```python
from build123d import *

# Parameters (mm, degrees)
Y_KSEKLIK_EKSTR_ZYON1_DEPTH = 40
BO_ALTMA1_START             = 2
BO_ALTMA1_DEPTH             = 36
IZIM4_W                     = 38.8
IZIM4_H                     = 1.5
KES_EKSTR_ZYON1_DEPTH       = 10
IZIM5_R                     = 1.45
IZIM5_R_2                   = 19
KES_EKSTR_ZYON2_DEPTH       = 2
IZIM6_W                     = 6.5
IZIM6_H                     = 6.5
IZIM6_R                     = 1.55
Y_KSEKLIK_EKSTR_ZYON2_DEPTH = 3
RADYUS1_R                   = 2
KES_EKSTR_ZYON3_DEPTH       = 10
KES_EKSTR_ZYON3_DEPTH_BACK  = 55


# Read off the part's stored shape, not the designer's step: İç Boşaltma1
with BuildPart() as part:
    # Çizim2 → Yükseklik-Ekstrüzyon1 (new body)
    with BuildSketch(Plane(origin=(0, 0, 0), x_dir=(0, 0, -1), z_dir=(1, 0, 0))):
        with BuildLine():
            Line((-8.520601237, 2.655177464), (-8.520601237, -7.344822536))
            ThreePointArc((-8.520601237, -7.344822536), (-8.2732007, -8.537800405), (-7.571803773, -9.53401603))
            Line((-7.571803773, -9.53401603), (-2.399280893, -14.708783566))
            ThreePointArc((-2.399280893, -14.708783566), (-1.426311448, -15.35897725), (-0.27796055, -15.587463223))
            Line((-0.27796055, -15.587463223), (-1.843021011, -18.19863418))
            add(Edge.make_bspline(
                [(-46.665907249, -13.909076506), (-24.516902354, -18.673937552), (-1.843021011, -18.19863418)],
                knots=[0, 0, 0, 1, 1, 1], degree=2))
            Line((-46.665907249, -13.909076506), (-46.665907249, -11.228578501))
            Line((-46.665907249, -11.228578501), (-8.520601237, 2.655177464))
        make_face()
    extrude(amount=Y_KSEKLIK_EKSTR_ZYON1_DEPTH)

    # İç Boşaltma1 outline → İç Boşaltma1 (cut)
    with BuildSketch(Plane.YZ.offset(BO_ALTMA1_START)):
        with BuildLine():
            Line((-0.201118549, 10.520601237), (-12.409947295, 44.064082645))
            add(Edge.make_bspline(
                [(-12.409947295, 44.064082645), (-12.786167702, 42.211926114), (-13.142061282, 40.357797151), (-13.477631026, 38.501688751), (-13.792879631, 36.643593797), (-14.087809503, 34.783505061), (-14.362422751, 32.921415207), (-14.616721192, 31.057316786), (-14.850706351, 29.19120224), (-15.064379456, 27.323063899), (-15.257741445, 25.452893983), (-15.526587368, 22.544304232), (-15.616158228, 21.507298941), (-15.699505521, 20.469667421), (-15.77662923, 19.431408364), (-15.847529338, 18.39252046), (-15.912205827, 17.353002403), (-15.970658681, 16.312852883), (-16.02288788, 15.272070593), (-16.06889341, 14.230654225), (-16.108675251, 13.18860247), (-16.159012454, 11.624569796), (-16.174235562, 11.103066399), (-16.187902686, 10.581403672), (-16.200013803, 10.059581454), (-16.210568888, 9.537599587), (-16.219567918, 9.01545791), (-16.227010868, 8.493156266), (-16.232897715, 7.970694494), (-16.237228434, 7.448072435), (-16.240003003, 6.92528993), (-16.241792402, 6.157267265), (-16.242021612, 5.912152435), (-16.241909023, 5.667002314), (-16.241454632, 5.421816888), (-16.240658436, 5.176596139), (-16.23952043, 4.931340051), (-16.238040611, 4.68604861), (-16.236218976, 4.440721798), (-16.234055521, 4.1953596), (-16.231550242, 3.949961999), (-16.228703137, 3.704528981)],
                knots=[0.04971795, 0.04971795, 0.04971795, 0.04971795, 0.04971795, 0.04971795, 0.04971795, 0.04971795, 0.04971795, 0.04971795, 0.04971795, 0.04971795, 0.513850496, 0.513850496, 0.513850496, 0.513850496, 0.513850496, 0.513850496, 0.513850496, 0.513850496, 0.513850496, 0.513850496, 0.770775744, 0.770775744, 0.770775744, 0.770775744, 0.770775744, 0.770775744, 0.770775744, 0.770775744, 0.770775744, 0.770775744, 0.899238368, 0.899238368, 0.899238368, 0.899238368, 0.899238368, 0.899238368, 0.899238368, 0.899238368, 0.899238368, 0.899238368, 0.959442934, 0.959442934, 0.959442934, 0.959442934, 0.959442934, 0.959442934, 0.959442934, 0.959442934, 0.959442934, 0.959442934, 0.959442934, 0.959442934], degree=11))
            ThreePointArc((-16.228703137, 3.704528981), (-16.17611264, 3.759568607), (-16.122690278, 3.81380118))
            Line((-16.122690278, 3.81380118), (-10.968143105, 8.966112527))
            ThreePointArc((-10.968143105, 8.966112527), (-9.316172777, 10.115574384), (-7.344822536, 10.520601237))
            Line((-7.344822536, 10.520601237), (-0.201118549, 10.520601237))
        make_face()
    extrude(amount=BO_ALTMA1_DEPTH, mode=Mode.SUBTRACT)

    # Çizim4 → Kes-Ekstrüzyon1 (cut)
    with BuildSketch(Plane(origin=(0, -3.997164066, -6.668930038), x_dir=(-1, 0, 0), z_dir=(0, -0.5140990756107078, -0.8577308088533464))):
        with Locations((-20, -15.0127467)):
            Rectangle(IZIM4_W, IZIM4_H)
    extrude(amount=-KES_EKSTR_ZYON1_DEPTH, mode=Mode.SUBTRACT)

    # Çizim5 → Kes-Ekstrüzyon2 (cut)
    with BuildSketch(Plane(origin=(0, 5.083049154, 1.850078591), x_dir=(1, 0, 0), z_dir=(0, 0.9396926207859106, 0.34202014332566266))):
        with Locations(Location((4, -11.159288927, 0), (0, 0, 270))):
            Circle(IZIM5_R)
        with Locations(Location((35.999942492, -11.09862193, 0), (0, 0, 270))):
            Circle(IZIM5_R)
        with Locations(Location((4, -43.159288927, 0), (0, 0, 270))):
            Circle(IZIM5_R)
        with Locations(Location((35.999942492, -43.09862193, 0), (0, 0, 270))):
            Circle(IZIM5_R)
        with Locations(Location((20, -27.798590964, 0), (0, 0, 270))):
            Circle(IZIM5_R_2)
    extrude(amount=-KES_EKSTR_ZYON2_DEPTH, mode=Mode.SUBTRACT)

    # Çizim6 → Yükseklik-Ekstrüzyon2 (add)
    # profile 1 of 2: a face of its own
    with BuildSketch(Plane(origin=(0, 0, 8.520601237), x_dir=(-1, 0, 0), z_dir=(0, 0, -1))):
        with Locations((-43.25, -0.594822536)):
            Rectangle(IZIM6_W, IZIM6_H)
        with Locations(Location((-43.25, -0.594822536, 0), (0, 0, 90))):
            Circle(IZIM6_R, mode=Mode.SUBTRACT)
    # profile 2 of 2: a face of its own
    with BuildSketch(Plane(origin=(0, 0, 8.520601237), x_dir=(-1, 0, 0), z_dir=(0, 0, -1))):
        with Locations((3.25, -0.594822536)):
            Rectangle(IZIM6_W, IZIM6_H)
        with Locations(Location((3.25, -0.594822536, 0), (0, 0, 90))):
            Circle(IZIM6_R, mode=Mode.SUBTRACT)
    extrude(amount=-Y_KSEKLIK_EKSTR_ZYON2_DEPTH)

    # Radyus1
    radyus1_edges = [part.edges().sort_by_distance(p)[0] for p in [
        (-6.5, -3.844822536, 10.020601237),
        (-6.5, 2.655177464, 10.020601237),
        (46.5, -3.844822536, 10.020601237),
        (46.5, 2.655177464, 10.020601237),
    ]]
    fillet(radyus1_edges, radius=RADYUS1_R)

    # Çizim7 → Kes-Ekstrüzyon3 (cut, two sides: drawn at the far end of the back side and taken through both)
    with BuildSketch(Plane.ZY.offset(-KES_EKSTR_ZYON3_DEPTH_BACK)):
        Polygon((11.520601237, 1.563266761), (8.520601237, 2.655177464), (11.520601237, 2.655177464), align=None)
    extrude(amount=KES_EKSTR_ZYON3_DEPTH + KES_EKSTR_ZYON3_DEPTH_BACK, mode=Mode.SUBTRACT)


solid = part.part
```
Model file for the job. Use its own axes, mm. A direction names the side the tool comes from. Give positions to 0.01 mm unless a question says otherwise; leave off trailing zeros. Loops run counter-clockwise (first coordinate to the right, second up) from the corner with the lowest first, then second, coordinate; pieces in that order, holes last. Notation, with made-up numbers: (74, -21.75) -> (92, -21.75) arc R21 ccw to (92, -1.75) -> close; hole circle Ø11 at (5, 61). An arc over 180 degrees is marked (long way). Write each question's results on one line, items separated by ' | '.
(1) Cut at A-A on x = -3.25. List the corners of the cut face in (y, z), and give its area (3 significant figures).
Geometry results:
outline: (-3.84, 8.52) -> (-2.14, 8.52) -> (-2.14, 11.52) -> (-3.84, 11.52) -> close; (0.96, 8.52) -> (2.66, 8.52) -> (1.56, 11.52) -> (0.96, 11.52) -> close | area: 8.56 mm²
(2) Tool access for faces 1 (the flat face through (-2, -3.845, 10)), 2 (the flat face through (42, -3.845, 10)), 3 (the flat face through (43.3, -2.3, 11.521)), 4 (the flat face through (38.71, -11.72, 9.62)): list every direction of +Z, -Z, +X, -X, +Y, -Y with a clear straight run to the whole face (end or side of a thin tool).
Geometry results:
face 1: +Z, -Z, -X, -Y | face 2: +Z, -Z, +X, -Y | face 3: +Z, +X, +Y, -Y | face 4: none
(3) Flat gauge pins, fed straight in: pin 1 Ø2.5 at (x, y) = (42.5, -2) entering from +Z; pin 2 Ø3.5 at (x, y) = (-3.25, -0.59) entering from -Z; pin 3 Ø5 at (y, z) = (-15, 6.5) entering from -X; pin 4 Ø1.9 at (x, y) = (43.25, -0.59) entering from -Z. Where does each tip first touch, or does it go through?
Geometry results:
pin 1: stops at z = 11.52 | pin 2: stops at z = 8.52 | pin 3: stops at x = 0 | pin 4: passes through
(4) Pull direction Y, two halves, no side cores. Call faces 5 (the flat face through (19.72, -17.745, 1.571)), 6 (the flat face through (20, -4, 10.521)), 7 (the flat face through (46.5, -1, 10)): released by +Y, released by -Y, zero draft, split by the parting line, or undercut.
Geometry results:
face 5: released by -Y | face 6: undercut | face 7: zero draft
(5) Probe line 1 along X through (y, z) = (-4.5, 14); line 2 along X through (y, z) = (0.25, 12); line 3 along X through (y, z) = (-14.5, 4.5). List the from-to ranges inside material, lowest first.
Geometry results:
line 1: x = 0 to 2, 38 to 40 | line 2: x = 0 to 2.55, 5.45 to 10.77, 29.23 to 34.55, 37.45 to 40 | line 3: x = 0 to 0.6, 39.4 to 40
